```python
from build123d import *

# Parameters (mm, degrees)
SKETCH1_R           = 20
BOSS_EXTRUDE1_DEPTH = 22.5
SKETCH2_R           = 3
BOSS_EXTRUDE2_DEPTH = 10
SKETCH3_R           = 1
CUT_EXTRUDE1_DEPTH  = 2
CIRPATTERN1_COUNT   = 6
CIRPATTERN1_ANGLE   = 335


with BuildPart() as part:
    # Sketch1 → Boss-Extrude1 (new body, symmetric)
    with BuildSketch(Plane.XY):
        Circle(SKETCH1_R)
    extrude(amount=BOSS_EXTRUDE1_DEPTH, both=True)

    # Sketch2 → Boss-Extrude2 (add)
    with BuildSketch(Plane.XY.offset(22.5)):
        Circle(SKETCH2_R)
    extrude(amount=BOSS_EXTRUDE2_DEPTH)

    # Sketch3 → Cut-Extrude1 (cut)
    with BuildSketch(Plane.XY.offset(22.5)):
        with Locations((0, 10)):
            Circle(SKETCH3_R)
    cut_extrude1 = extrude(amount=-CUT_EXTRUDE1_DEPTH, mode=Mode.SUBTRACT)

    # CirPattern1: Cut-Extrude1 ×6 about axis
    cirpattern1_axis = Axis((0, 0, 0), (0, 0, -1))
    for i in range(1, CIRPATTERN1_COUNT):
        add(cut_extrude1.rotate(cirpattern1_axis, i * CIRPATTERN1_ANGLE / (CIRPATTERN1_COUNT - 1)), mode=Mode.SUBTRACT)


solid = part.part
```
Design review of the part built by this model. Coordinates are the model's own, in mm. A direction names the side the tool comes from. Round coordinates to 2 decimals unless told otherwise and drop trailing zeros. Order: outer loops, then holes, each group sorted by start corner. A loop starts at its lowest first (then second) coordinate and runs counter-clockwise, first axis right, second up. Notation, with made-up numbers: (18.25, 80) - (76.25, 80) arc R18 ccw to (76.25, 88) - close; hole circle Ø7 at (77.25, 9.5). An arc over 180 degrees is marked (long way). Return JSON: item names as keys, results as strings.
Q1. The part is to be moulded in two halves that separate along X. For faces 1 (the flat face through (-10, 0, 20.5)), 2 (the cylindrical face through (-4.336, -19.524, 0.315)), 3 (the flat face through (0, 0, 32.5)), say which applies: pulls with the +X half, pulls with the -X half, needs draft (parallel to the pull), parting line crosses it, or undercut.
Computed values:
{"face 1": "undercut", "face 2": "parting line crosses it", "face 3": "needs draft"}
Q2. Consider section B-B on y = 0. Write out the cut boundary in (x, z), plus the area to 3 significant figures.
Computed values:
{"outline": "(-20, -22.5) - (20, -22.5) - (20, 22.5) - (3, 22.5) - (3, 32.5) - (-3, 32.5) - (-3, 22.5) - (-9.06, 22.5) - (-9.06, 20.5) - (-10.93, 20.5) - (-10.93, 22.5) - (-20, 22.5) - close", "area": "1,860 mm2"}
Q3. Machinability: for faces 4 (the cylindrical face through (-3, 0, 27)), 5 (the flat face through (0, 0, -22.5)), which of the approach directions +Z, -Z, +X, -X, +Y, -Y give a long, thin tool a straight path to every point of the face, cutting with its end or side? Answer none if there is none.
Computed values:
{"face 4": "+Z", "face 5": "-Z, +X, -X, +Y, -Y"}
Q4. Consider section C-C on z = 5. Write out the cut boundary in (x, y).
Computed values:
{"outline": "circle Ø40 at (0, 0)"}
Q5. For pin 1 Ø1 at (x, y) = (-3.5, -9) entering from +Z; pin 2 Ø12 at (y, z) = (11, -9) entering from -X; pin 3 Ø1 at (y, z) = (-2.5, 10.5) entering from -X; pin 4 Ø10 at (y, z) = (2.5, -14.5) entering from +X, all flat-tipped, find the tip position at first contact; note any pin that passes through.
Computed values:
{"pin 1": "stops at z = 20.5", "pin 2": "stops at x = -19.36", "pin 3": "stops at x = -19.9", "pin 4": "stops at x = 20"}
Q6. Consider section A-A on x = 0. Write out the cut boundary in (y, z).
Computed values:
{"outline": "(-20, -22.5) - (20, -22.5) - (20, 22.5) - (11, 22.5) - (11, 20.5) - (9, 20.5) - (9, 22.5) - (3, 22.5) - (3, 32.5) - (-3, 32.5) - (-3, 22.5) - (-20, 22.5) - close"}
Q7. Wall thickness on L1, parallel to Z at x = 1, y = 6; L2, parallel to Y at x = -18, z = 3; L3, parallel to X at y = 15.5, z = -9: over which ranges is each line inside the solid? List them lowest first. Write a range as [from, to].
Computed values:
{"L1": "z = [-22.5, 22.5]", "L2": "y = [-8.72, 8.72]", "L3": "x = [-12.64, 12.64]"}
Q8. Consider section D-D on y = 12. Write out the cut boundary in (x, z).
Computed values:
{"outline": "(-16, -22.5) - (16, -22.5) - (16, 22.5) - (-16, 22.5) - close"}
